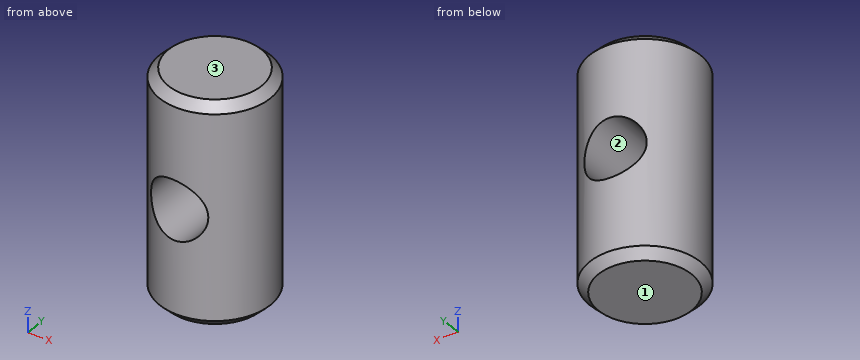
from build123d import *

# Parameters (mm, degrees)
SKETCH1_R               = 4.765
BOSS_EXTRUDE1_DEPTH     = 9.525
CHAMFER1_SIZE           = 0.76
CUT_EXTRUDE1_DEPTH      = 12.667736499
CUT_EXTRUDE1_DEPTH_BACK = 12.667736499
SKETCH2_R               = 2.555


with BuildPart() as part:
    # Sketch1 → Boss-Extrude1 (new, symmetric)
    with BuildSketch(Plane.XY):
        with Locations(Location((0, 0, 0), (0, 0, 180))):
            Circle(SKETCH1_R)
    extrude(amount=BOSS_EXTRUDE1_DEPTH, both=True)

    # Chamfer1
    chamfer1_edges = [part.edges().sort_by_distance(p)[0] for p in [
        (4.765, 0, -9.525),
        (4.765, 0, 9.525),
    ]]
    chamfer(chamfer1_edges, length=CHAMFER1_SIZE)

    # Sketch2 → Cut-Extrude1 (cut, two sides: drawn at the far end of the back side and taken through both)
    with BuildSketch(Plane(origin=(0, 0, 0), x_dir=(1, 0, 0), z_dir=(0, 1, 0)).offset(-CUT_EXTRUDE1_DEPTH_BACK)):
        with Locations(Location((-0.25, 0, 0), (0, 0, 270))):
            Circle(SKETCH2_R)
    extrude(amount=CUT_EXTRUDE1_DEPTH + CUT_EXTRUDE1_DEPTH_BACK, mode=Mode.SUBTRACT)


solid = part.part
Part model, mm, in its own coordinate system. Face numbers are marked on the shaded views. Coordinates: 2 decimals unless noted, no trailing zeros. Write each loop counter-clockwise with the first axis right and the second up, starting at its lowest first coordinate (ties: lowest second). Pieces come first, ordered by that corner, then holes. Notation, with made-up numbers: (42.5, 9.25) - (47.5, 9.25) arc R9 ccw to (47.5, 13.25) - close; hole circle Ø1 at (65.5, 81). An arc over 180 degrees is marked (long way). Put each result on its own line as item: value.
1. Band-saw the part on D-D (z = -6.75). Write the cut outline in (x, y) (3 decimals), then the cut area to 3 significant figures.
Final values:
outline: circle Ø9.53 at (0, 0)
area: 71.3 mm²
2. Flat gauge pins, fed straight in: pin 1 Ø1 at (x, z) = (-1, 5.5) entering from -Y; pin 2 Ø3 at (x, z) = (-0.25, 0) entering from -Y; pin 3 Ø1.5 at (y, z) = (-1, -7.5) entering from +X. Where does each tip first touch, or does it go through?
Final values:
pin 1: stops at y = -4.74
pin 2: passes through
pin 3: stops at x = 4.76
3. Band-saw the part on B-B (x = 0). Write the cut outline in (y, z) (3 decimals), then the cut area to 3 significant figures.
Final values:
outline: (-4.765, -8.765) - (-4.005, -9.525) - (4.005, -9.525) - (4.765, -8.765) - (4.765, -2.543) - (-4.765, -2.543) - close; (-4.765, 2.543) - (4.765, 2.543) - (4.765, 8.765) - (4.005, 9.525) - (-4.005, 9.525) - (-4.765, 8.765) - close
area: 132 mm²
4. Probe line 1 along Z through (x, y) = (-0.25, 1.75) (3 decimals); line 2 along X through (y, z) = (2, 1); line 3 along Z through (x, y) = (-0.75, 3.75) (3 decimals). List the from-to ranges inside material, lowest first. Write a range as [from, to].
Final values:
line 1: z = [-9.525, -2.555], [2.555, 9.525]
line 2: x = [-4.32, -2.6], [2.1, 4.32]
line 3: z = [-9.525, -2.506], [2.506, 9.525]
5. Two-plate mould, pull along Z, no slides. Class the marked faces 1, 2 and 3: +Z half, -Z half, draft (parallel to the pull), parting line (faces both ways), or undercut.
Final values:
face 1: -Z half
face 2: undercut
face 3: +Z half
6. Band-saw the part on A-A (y = 0). Write the cut outline in (x, z) (3 decimals).
Final values:
outline: (-4.765, -8.765) - (-4.005, -9.525) - (4.005, -9.525) - (4.765, -8.765) - (4.765, 8.765) - (4.005, 9.525) - (-4.005, 9.525) - (-4.765, 8.765) - close; hole circle Ø5.11 at (-0.25, 0)
7. Band-saw the part on C-C (z = 0). Write the cut outline in (x, y) (3 decimals).
Final values:
outline: (-2.805, -3.852) - (-2.805, 3.852) arc R4.765 ccw to start; (2.305, -4.17) arc R4.765 ccw to (2.305, 4.17) - close
